Source: CAD feature listing. Evaluate the final solid. Frame: model axes, mm. A direction names the side the tool comes from. Give positions to 0.01 mm unless a question says otherwise; leave off trailing zeros. Write each loop counter-clockwise with the first axis right and the second up, starting at its lowest first coordinate (ties: lowest second). Pieces come first, ordered by that corner, then holes. Notation, with made-up numbers: (42.25, -3) -> (95.25, -3) arc R6 ccw to (95.25, 2) -> close; hole circle Ø8 at (29, 55.25). An arc over 180 degrees is marked (long way). Use a Markdown table: item, result. Add a question column.
```python
from build123d import *

# Parameters (mm, degrees)
F0_R     = 19.05
F1_DEPTH = 152.4
F2_R     = 14.2875
F3_DEPTH = 3.175
F4_R     = 19.05
F5_DEPTH = 3.175


with BuildPart() as f1:
    # F0 (on Top) → F1 (new body)
    with BuildSketch(Plane.XY):
        Circle(F0_R)
    extrude(amount=-F1_DEPTH)

    # F2 (on face) → F3 (join)
    with BuildSketch(Plane.XY):
        Circle(F2_R)
    extrude(amount=F3_DEPTH)

    # F4 (on face) → F5 (join)
    with BuildSketch(Plane.XY.offset(3.175)):
        Circle(F4_R)
    extrude(amount=F5_DEPTH)


solid = f1.part
```
(1) Material intervals for L1, parallel to Z at x = -6.5, y = 13.5 (3 decimals); L2, parallel to Y at x = 0.5, z = -49.5; L3, parallel to X at y = -15.5, z = -32, sorted ascending.
(2) Cut plane B-B on z = -82. Return the cut outline in (x, y), then the cut area to 3 significant figures.
(3) First-contact query: pin 1 Ø10 at (x, z) = (-4, -32) entering from +Y; pin 2 Ø6 at (y, z) = (-3.5, -103) entering from +X; pin 3 Ø5 at (x, z) = (0, -83) entering from -Y; pin 4 Ø12 at (y, z) = (-3, -114.5) entering from -X. Flat tips, straight axial feed; report the tip coordinate or a pass-through.
(4) Access query for faces 1 (the flat face through (0, 0, -152.4)), 2 (the cylindrical face through (-14.274, 0.628, 1.565)). Directions: +Z, -Z, +X, -X, +Y, -Y. A direction counts if a zero-diameter tool reaches every point of the face in a straight line with its end or side. Return the directions, or none.
(5) Cut plane A-A on y = 5.5. Return the cut outline in (x, z) (3 decimals).
(6) Mould query, pull axis Z, two halves, no side actions, for faces 3 (the flat face through (0, 0, 6.35)), 4 (the flat face through (2.7, 14.2, 3.175)), 5 (the cylindrical face through (-15.12, -11.59, 4.74)). Classes: +Z half, -Z half, draft (parallel to the pull), parting line (faces both ways), or undercut.
(7) Cut plane C-C on x = 8. Return the cut outline in (y, z) (3 decimals), then the cut area to 3 significant figures.
Output:
| question | item | result |
|---|---|---|
| 1 | L1 | -152.4 to 0, 3.175 to 6.35 |
| 1 | L2 | -19.04 to 19.04 |
| 1 | L3 | -11.07 to 11.07 |
| 2 | outline | circle Ø38.1 at (0, 0) |
| 2 | area | 1,140 mm^2 |
| 3 | pin 1 | y = 19.05 |
| 3 | pin 2 | x = 19.04 |
| 3 | pin 3 | y = -19.05 |
| 3 | pin 4 | x = -19.05 |
| 4 | face 1 | -Z, +X, -X, +Y, -Y |
| 4 | face 2 | none |
| 5 | outline | (-18.239, -152.4) -> (18.239, -152.4) -> (18.239, 0) -> (13.186, 0) -> (13.186, 3.175) -> (18.239, 3.175) -> (18.239, 6.35) -> (-18.239, 6.35) -> (-18.239, 3.175) -> (-13.186, 3.175) -> (-13.186, 0) -> (-18.239, 0) -> close |
| 6 | face 3 | +Z half |
| 6 | face 4 | undercut |
| 6 | face 5 | draft |
| 7 | outline | (-17.289, -152.4) -> (17.289, -152.4) -> (17.289, 0) -> (11.838, 0) -> (11.838, 3.175) -> (17.289, 3.175) -> (17.289, 6.35) -> (-17.289, 6.35) -> (-17.289, 3.175) -> (-11.838, 3.175) -> (-11.838, 0) -> (-17.289, 0) -> close |
| 7 | area | 5,450 mm^2 |
